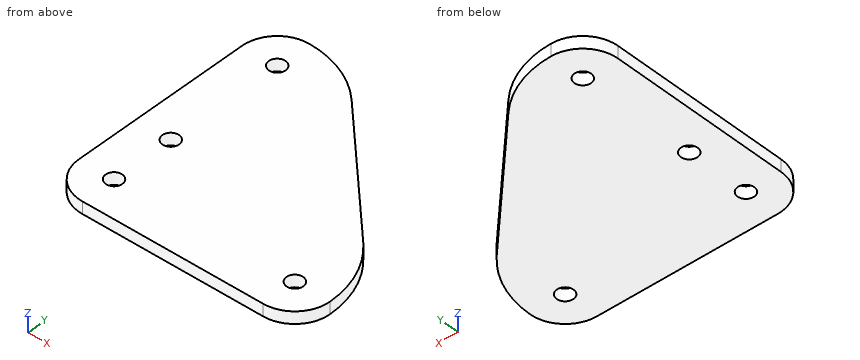
```python
from build123d import *

# Parameters (mm, degrees)
BOSS_EXTRUDE1_DEPTH      = 3
FILLET1_R                = 21.5
FILLET2_R                = 52
CUT_EXTRUDE1_DEPTH       = 189.18607812481773
F_5_16_CLEARANCE_HOLE1_D = 8.3185


with BuildPart() as part:
    # Sketch1 → Boss-Extrude1 (new, symmetric)
    with BuildSketch(Plane.XY):
        Polygon((0, 0), (0, 133), (42.999999999999986, 133), (133, 42.99999999999999), (133, 9.06e-15), align=None)
    extrude(amount=BOSS_EXTRUDE1_DEPTH, both=True)

    # Fillet1
    fillet1_edges = [part.edges().sort_by_distance(p)[0] for p in [
        (0, 0, 0),
        (0, 133, 0),
        (133, 9.06e-15, 0),
    ]]
    fillet(fillet1_edges, radius=FILLET1_R)

    # Fillet2
    # the kernel refuses this fillet: 52 mm, written as the material it takes off along each edge
    with BuildSketch(Plane(origin=(133, 43, -56.84767436170304), x_dir=(-0.7071067811865476, 0.7071067811865476, 0), z_dir=(0, 0, 1))) as fillet2_piece_1:
        with BuildLine():
            CenterArc((21.539069744681207, 52.00000000000001), FILLET2_R, 225.07350833515432, 44.926491664845685)
            Line((-15.183278672480162, 15.183303696167892), (-18.855513514196304, 11.501634065784673))
            ThreePointArc((-18.855513514196304, 11.501634065784673), (-18.87975105768081, 11.52584053334073), (-3.6769552621700394, -3.6769552621700394))
            Line((-3.6769552621700394, -3.6769552621700394), (-4.9e-15, -5.200000000000005))
            Line((-4.9e-15, -5.200000000000005), (21.539069744681218, -5.199999999999996))
            Line((21.539069744681218, -5.199999999999996), (21.539069744681214, 4.7e-16))
        make_face()
    extrude(amount=113.69534872340608, mode=Mode.SUBTRACT)
    with BuildSketch(Plane(origin=(42.999999999999986, 133, 56.847674361702985), x_dir=(-0.9999999999996605, -8.240534738615283e-07, 0), z_dir=(0, 0, -1))) as fillet2_piece_2:
        with BuildLine():
            CenterArc((21.539173195539043, -51.9999571492017), FILLET2_R, 90.07355554994047, 44.926491664845685)
            Line((-15.230409726226513, -15.230434827591285), (-18.90736801840307, -11.55348259543025))
            Line((-18.90736801840307, -11.55348259543025), (-3.676958292176556, 3.6769522321610486))
            Line((-3.676958292176556, 3.6769522321610486), (-4.28507806408e-06, 5.199999999998223))
            ThreePointArc((-4.28507806408e-06, 5.199999999998223), (21.499995714914625, 5.200017717147912), (21.46574062621809, 5.1999957149201785))
            Line((21.46574062621809, 5.1999957149201785), (21.472416314338172, 0))
        make_face()
    extrude(amount=113.69534872340597, mode=Mode.SUBTRACT)

    # Sketch3 → Cut-Extrude1 (cut, through all)
    with BuildSketch(Plane.XY.offset(3)):
        with BuildLine():
            Line((117.76956733680983, 58.23043266319015), (58.23043266319017, 117.76956733680981))
            ThreePointArc((58.23043266319017, 117.76956733680981), (41.3784881824358, 129.03426172642116), (21.499999999999996, 133))
            ThreePointArc((21.499999999999996, 133), (6.2972042044892405, 126.70279579551078), (3.47e-15, 111.50000000000001))
            Line((3.47e-15, 111.50000000000001), (0, 21.5))
            ThreePointArc((0, 21.5), (6.297204204489223, 6.297204204489235), (21.49999999999999, 3.47e-15))
            Line((21.49999999999999, 3.47e-15), (111.50000000000001, 1.041e-14))
            ThreePointArc((111.50000000000001, 1.041e-14), (126.70279579551078, 6.297204204489239), (133, 21.500000000000007))
            ThreePointArc((133, 21.500000000000007), (129.03426172642114, 41.37848818243579), (117.76956733680983, 58.23043266319015))
        make_face()
        with BuildLine():
            Line((114.94114021206362, 55.40200553844396), (55.402005538443966, 114.94114021206363))
            ThreePointArc((55.402005538443966, 114.94114021206363), (39.84708125964561, 125.33902242576387), (21.49854269401705, 128.9999999393217))
            ThreePointArc((21.49854269401705, 128.9999999393217), (9.12511610449009, 123.87385342456624), (4.0000000000000036, 111.50000000000001))
            Line((4.0000000000000036, 111.50000000000001), (4, 21.500000000000004))
            ThreePointArc((4, 21.500000000000004), (9.125631329235414, 9.125631329235425), (21.499999999999996, 4.0000000000000036))
            Line((21.499999999999996, 4.0000000000000036), (111.50000000000001, 4.000000000000011))
            ThreePointArc((111.50000000000001, 4.000000000000011), (123.8738534245646, 9.125116104488455), (128.9999999393217, 21.49854269401244))
            ThreePointArc((128.9999999393217, 21.49854269401244), (125.33902242576474, 39.847081259643474), (114.94114021206362, 55.40200553844396))
        make_face(mode=Mode.SUBTRACT)
    extrude(amount=-CUT_EXTRUDE1_DEPTH, mode=Mode.SUBTRACT)


with BuildPart() as cut_extrude1_kept_piece:
    # of the separate pieces the step leaves, the one the design keeps (cut_extrude1_pieces_kept)
    add(part.part.solids().sort_by_distance((128.999999939, 21.498542694, -3))[0])

    # 5/16 Clearance Hole1 (through all)
    with Locations(Plane.XY.offset(3)):
        with Locations((21.5, 111.5), (21.5, 52.7884), (21.5, 21.5), (111.5, 21.5)):
            Hole(F_5_16_CLEARANCE_HOLE1_D / 2)


solid = cut_extrude1_kept_piece.part
```
Here's how the part is built. I have some questions about the finished solid (model axes, mm). Give positions to 0.01 mm unless a question says otherwise; leave off trailing zeros. Order: outer loops, then holes, each group sorted by start corner. A loop starts at its lowest first (then second) coordinate and runs counter-clockwise, first axis right, second up. Notation, with made-up numbers: (-17, -28) -> (-5, -28) arc R37 cw to (-5, 11) -> close; hole circle Ø6 at (58, 60). An arc over 180 degrees is marked (long way). Use CSV: the item, a comma, the result in double quotes. Start each with the question number.
Item 1: I'm going to push flat-ended pins straight in: P1, Ø13.5, axis at x = 21.5, y = 111.5, coming from the +Z side; P2, Ø2, axis at y = 62, z = 0, coming from the +X side; P3, Ø1, axis at x = 111.5, z = -0.5, coming from the +Y side. Where does each tip first touch, or does it pass through?
Item 2: Suppose I cut it at D-D (x = 70). List the corners of the cut face in (y, z) for me.
Item 3: Suppose I cut it at B-B (y = 23.5). List the corners of the cut face in (x, z) for me, and give its area (3 significant figures).
Item 4: Suppose I cut it at C-C (y = 113). List the corners of the cut face in (x, z) for me.
Item 5: Suppose I cut it at A-A (z = -0.8). List the corners of the cut face in (x, y) for me.
Item 6: If I drill on probe 1 along Y at (x, z) = (21.5, -0.9); probe 2 along X at (y, z) = (109, -2.25); probe 3 along Y at (x, z) = (87.5, -2.6), over which ranges is the centre line in solid material (lowest first)? Write a range as [from, to].
Answer block:
1,P1,"stops at z = 3"
1,P2,"stops at x = 109.34"
1,P3,"stops at y = 59.34"
2,outline,"(4, -3) -> (100.34, -3) -> (100.34, 3) -> (4, 3) -> close"
3,outline,"(4, -3) -> (17.85, -3) -> (17.85, 3) -> (4, 3) -> close; (25.15, -3) -> (107.85, -3) -> (107.85, 3) -> (25.15, 3) -> close; (115.15, -3) -> (128.96, -3) -> (128.96, 3) -> (115.15, 3) -> close"
3,area,"662 mm^2"
4,outline,"(4.06, -3) -> (17.62, -3) -> (17.62, 3) -> (4.06, 3) -> close; (25.38, -3) -> (57.34, -3) -> (57.34, 3) -> (25.38, 3) -> close"
5,outline,"(4, 21.5) arc R17.5 ccw to (21.5, 4) -> (111.5, 4) arc R17.5 ccw to (129, 21.5) arc R48 ccw to (114.94, 55.4) -> (55.4, 114.94) arc R48 ccw to (21.5, 129) arc R17.5 ccw to (4, 111.5) -> close; hole circle Ø8.32 at (21.5, 21.5); hole circle Ø8.32 at (21.5, 52.79); hole circle Ø8.32 at (21.5, 111.5); hole circle Ø8.32 at (111.5, 21.5)"
6,probe 1,"y = [4, 17.34], [25.66, 48.63], [56.95, 107.34], [115.66, 129]"
6,probe 2,"x = [4, 18.18], [24.82, 61.34]"
6,probe 3,"y = [4, 82.84]"
